Autodesk Inventor part; units mm, degrees
ref_plane "YZ Plane" through (0, 0, 0) normal (1, 0, 0) x (0, 1, 0)
ref_plane "XZ Plane" through (0, 0, 0) normal (0, 1, 0) x (-1, 0, 0)
ref_plane "XY Plane" through (0, 0, 0) normal (0, 0, 1) x (1, 0, 0)
sketch "Sketch1" plane through (0, 0, 0) normal (0, 0, 1) x (1, 0, 0)
  line L0 (-41.5, 50) -> (41.5, 50)
  line L1 (41.5, 50) -> (41.5, -50)
  line L2 (41.5, -50) -> (-41.5, -50)
  line L3 (-41.5, -50) -> (-41.5, 50)
  line L4 (35.5, 44) -> (-35.5, 44)
  line L5 (-35.5, 44) -> (-35.5, -44)
  line L6 (-35.5, -44) -> (35.5, -44)
  line L7 (35.5, -44) -> (35.5, 44)
  line L8 (-41.5, -47) -> (41.5, -47) construction
  circle A0 centre (-19.75, -47) radius 2.25
  line L9 (0, 71.7466) -> (0, -78.0681) construction
  circle A1 centre (0, -47) radius 2.25
  circle A2 centre (19.75, -47) radius 2.25
  line L10 (-60.2597, 0) -> (74.2823, 0) construction
  line L11 (-38.5, 50) -> (-38.5, -50) construction
  circle A3 centre (-38.5, 0) radius 2.25
  circle A4 centre (-38.5, 27) radius 2.25
  circle A5 centre (-38.5, -27) radius 2.25
  line L12 (-41.5, 47) -> (41.5, 47) construction
  line L13 (-35.5, -3) -> (-35.5, 3)
  circle A6 centre (-38.5, 47) radius 2.25
  circle A7 centre (-38.5, -47) radius 2.25
  line L14 (-25, 50) -> (25, 50)
  line L15 (25, 50) -> (25, 47)
  line L16 (25, 47) -> (-25, 47)
  line L17 (-25, 47) -> (-25, 50)
  circle A8 centre (-28, 47) radius 2.25
  circle A9 centre (28, 47) radius 2.25
  point P0 (0, 0)
  point P1 (0, 50)
  point P2 (41.5, 0)
  point P3 (0, 47)
  point P4 (0, 47)
  dimension "d0" = 83
  dimension "d1" = 100
  dimension "d2" = 4.5
  dimension "d3" = 4.5
  dimension "d4" = 4.5
  dimension "d5" = 3
  dimension "d6" = 3
  dimension "d9" = 3
  dimension "d10" = 4.5
  dimension "d11" = 4.5
  dimension "d12" = 4.5
  dimension "d17" = 3
  dimension "d41" = 4.5
  dimension "d42" = 4.5
  dimension "d45" = 29.25
  dimension "d46" = 29.25
  dimension "d47" = 22
  dimension "d48" = 22
  dimension "d66" = 50
  dimension "d67" = 3
  dimension "d81" = 4.5
  dimension "d82" = 4.5
  dimension "d83" = 3
  dimension "d84" = 3
extrude "Extrusion1" add sketch "Sketch1" along normal blind 1.5 contours L0 L17 L16 L15 L1 L2 L3 | L0 L15 L16 L17 | A3 | A4 | A5 | A6 | A7 | A8 | A9
extrude "Extrusion2" cut sketch "Sketch1" along normal blind 10 contours A3 | A4 | A5 | A6 | A7
mirror "Mirror1" about plane through (0, 0, 0) normal (1, 0, 0) of "Extrusion2"
extrude "Extrusion7" cut sketch "Sketch1" along normal blind 10 contours A8 | A9
properties part number "Side" material "ABS Plastic"
Design review of the part built by this model. Coordinates are the model's own, in mm. Coordinates: 2 decimals unless noted, no trailing zeros. Order: outer loops, then holes, each group sorted by start corner. A loop starts at its lowest first (then second) coordinate and runs counter-clockwise, first axis right, second up. Notation, with made-up numbers: (29.5, -23.5) - (52.5, -23.5) arc R24 cw to (52.5, -0.5) - close; hole circle Ø10 at (17.25, 75.25). An arc over 180 degrees is marked (long way). Answer in a Markdown table with one row per item.
(1) Consider section D-D on y = -35. State the section outline as (x, z) points, plus the area to 3 significant figures.
Checked values:
| item | result |
|---|---|
| outline | (-41.5, 0) - (-35.5, 0) - (-35.5, 1.5) - (-41.5, 1.5) - close; (35.5, 0) - (41.5, 0) - (41.5, 1.5) - (35.5, 1.5) - close |
| area | 18.0 mm^2 |
(2) Consider section C-C on z = 0.85. Give the number of separate pieces and of enclosed holes in the cut face, plus the area to 3 significant figures.
Checked values:
| item | result |
|---|---|
| separate pieces | 1 |
| enclosed holes | 16 |
| area | 1,810 mm^2 |
(3) Clearance check with flat-ended pins moving along their axes: pin 1 (7 mm diameter, centred on x = -38.5, y = -27, fed in from -Z); pin 2 (3.5 mm diameter, centred on x = -19.75, y = -47, fed in from +Z). State where each tip first meets the part, or that it passes through.
Checked values:
| item | result |
|---|---|
| pin 1 | z = 0 |
| pin 2 | through |
(4) Wall thickness on line 1 along Y through (x, z) = (38.5, 0.65); line 2 along Y through (x, z) = (12.5, 1.05); line 3 along X through (y, z) = (4, 1.3): over which ranges is each line inside the solid? List them lowest first. Write a range as from..to.
Checked values:
| item | result |
|---|---|
| line 1 | -50..-49.25, -44.75..-29.25, -24.75..-2.25, 2.25..24.75, 29.25..44.75, 49.25..50 |
| line 2 | -50..-44, 44..50 |
| line 3 | -41.5..-35.5, 35.5..41.5 |
(5) Consider section A-A on x = 0. State the section outline as (y, z) points.
Checked values:
| item | result |
|---|---|
| outline | (-50, 0) - (-49.25, 0) - (-49.25, 1.5) - (-50, 1.5) - close; (-44.75, 0) - (-44, 0) - (-44, 1.5) - (-44.75, 1.5) - close; (44, 0) - (50, 0) - (50, 1.5) - (44, 1.5) - close |
(6) The part is to be moulded in two halves that separate along X. For faces 1 (the flat face through (-37, 4, 0)), 2 (the cylindrical face through (29.21, 45.103, 0.74)), say which applies: released by +X, released by -X, zero draft, split by the parting line, or undercut.
Checked values:
| item | result |
|---|---|
| face 1 | zero draft |
| face 2 | undercut |
(7) Consider section B-B on y = -47. State the section outline as (x, z) points, plus the area to 4 significant figures.
Checked values:
| item | result |
|---|---|
| outline | (-41.5, 0) - (-40.75, 0) - (-40.75, 1.5) - (-41.5, 1.5) - close; (-36.25, 0) - (-22, 0) - (-22, 1.5) - (-36.25, 1.5) - close; (-17.5, 0) - (-2.25, 0) - (-2.25, 1.5) - (-17.5, 1.5) - close; (2.25, 0) - (17.5, 0) - (17.5, 1.5) - (2.25, 1.5) - close; (22, 0) - (36.25, 0) - (36.25, 1.5) - (22, 1.5) - close; (40.75, 0) - (41.5, 0) - (41.5, 1.5) - (40.75, 1.5) - close |
| area | 90.75 mm^2 |
